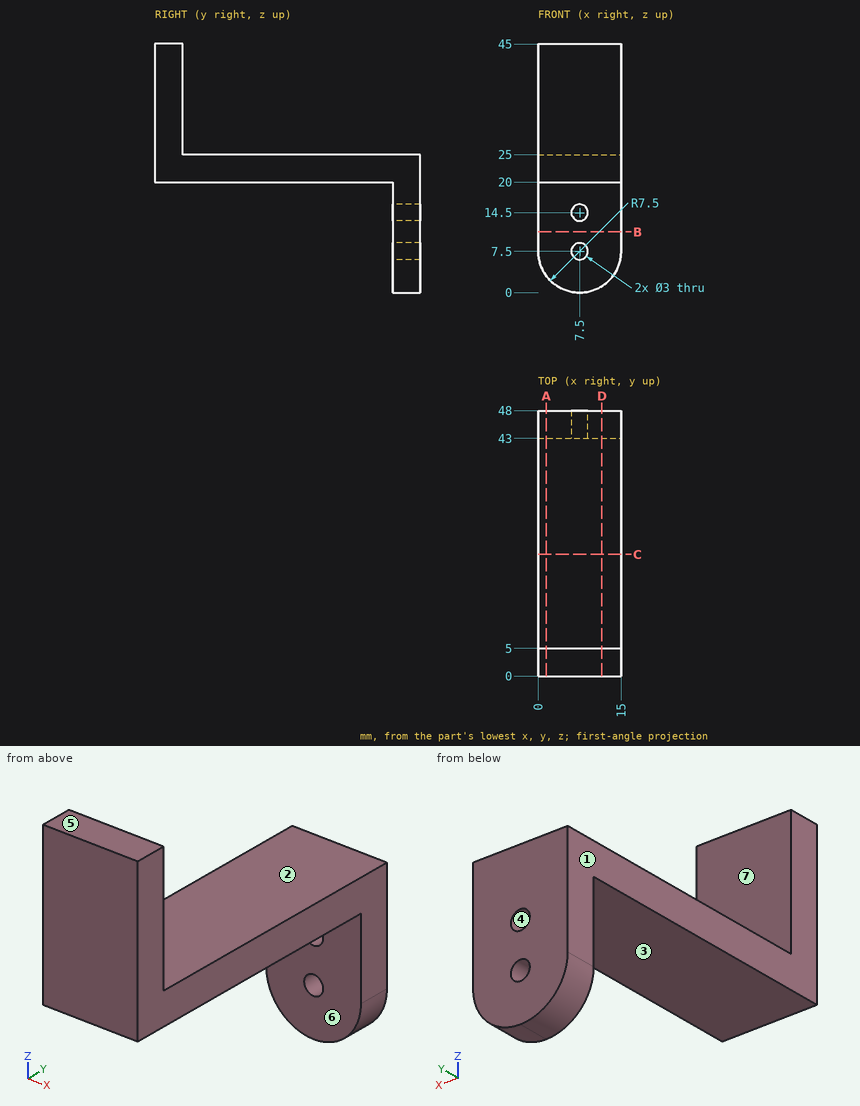
Verification items for this drawing (mm, ordinates from the low corner). A direction names the side the tool comes from. Give positions to 0.01 mm unless a question says otherwise; leave off trailing zeros. Loops run counter-clockwise (first coordinate to the right, second up) from the corner with the lowest first, then second, coordinate; pieces in that order, holes last.
1. Release check for a two-part mould opening along Z. For the marked faces 1, 2, 3 and 4 record: +Z half, -Z half, draft (parallel to the pull), parting line (faces both ways), or undercut.
Derived:
face 1: draft
face 2: +Z half
face 3: -Z half
face 4: undercut
2. Cross-section at A-A on x = 1.5. Record the cut outline in (y, z).
Derived:
outline: (0, 20) - (43, 20) - (43, 3) - (48, 3) - (48, 25) - (5, 25) - (5, 45) - (0, 45) - close
3. Go/stop test with flat-tipped pins: P1, Ø3, axis at x = 4, z = 27, coming from the +Y side; P2, Ø3, axis at x = 12, y = 9.5, coming from the -Z side; P3, Ø7.5, axis at x = 10.5, y = 17.5, coming from the +Z side. Record where each tip stops, or that it passes through.
Derived:
P1: stops at y = 5
P2: stops at z = 20
P3: stops at z = 25
4. Cross-section at B-B on z = 11. Record the cut outline in (x, y), and give its area (3 significant figures).
Derived:
outline: (0, 43) - (15, 43) - (15, 48) - (0, 48) - close
area: 75.0 mm2
5. Material ranges on probe 1 along Z at (x, y) = (13, 9.5); probe 2 along Y at (x, z) = (5, 42); probe 3 along Y at (x, z) = (6.25, 16.5), recorded low to high.
Derived:
probe 1: z = 20 to 25
probe 2: y = 0 to 5
probe 3: y = 43 to 48
6. Cross-section at D-D on x = 11.5. Record the cut outline in (y, z).
Derived:
outline: (0, 20) - (43, 20) - (43, 1.16) - (48, 1.16) - (48, 25) - (5, 25) - (5, 45) - (0, 45) - close
7. Tool access check on the marked faces 5, 6 and 7. Record the directions out of +Z, -Z, +X, -X, +Y, -Y that give a thin tool (end or side, any length) a straight path to the whole face; none if there is none.
Derived:
face 5: +Z, +X, -X, +Y, -Y
face 6: -Z, +X, -X, -Y
face 7: +Z, +X, -X, +Y
8. Cross-section at C-C on y = 22. Record the cut outline in (x, z), and give its area (3 significant figures).
Derived:
outline: (0, 20) - (15, 20) - (15, 25) - (0, 25) - close
area: 75.0 mm2
